CAD build for the part. Positions are in the model's coordinates, mm. A direction names the side the tool comes from. Give positions to 0.01 mm unless a question says otherwise; leave off trailing zeros. Order: outer loops, then holes, each group sorted by start corner. A loop starts at its lowest first (then second) coordinate and runs counter-clockwise, first axis right, second up.
Item 1: Flat gauge pins, fed straight in: P1, Ø1, axis at x = -50.5, z = 1, coming from the -Y side; P2, Ø5, axis at x = -38, y = -9, coming from the -Z side; P3, Ø0.9, axis at x = -24.5, z = 1, coming from the -Y side. Where does each tip first touch, or does it go through?
Item 2: Band-saw the part on B-B on y = -8.5. Give the cut face in (x, z), plus the area to 3 significant figures.
Item 3: Band-saw the part on D-D on y = -0.5. Give the cut face in (x, z), plus the area to 3 significant figures.
Item 4: Band-saw the part on A-A on x = -39. Give the cut face in (y, z), plus the area to 3 significant figures.
Item 5: Band-saw the part on C-C on z = 1.6. Give the cut face in (x, y), plus the area to 3 significant figures.
Item 6: Which spindle directions (+Z, -Z, +X, -X, +Y, -Y) get a long thin tool onto all of the face, cutting with end or side? Do faces 1 (the cylindrical face through (-51.5, -0.07, 1.48)), 2 (the flat face through (-30, 4.5, 1)), 3 (the flat face through (-30, -4.5, 1)). Say none if no direction does.
Item 7: Two-plate mould, pull along Y, no slides. Class faces 4 (the flat face through (-56.623, -1.288, 1.479)), 5 (the cylindrical face through (-40.2, -0.9, 1.5)), 6 (the cylindrical face through (-7.5, 0.1, 1.5)), 7 (the cylindrical face through (-59.277, -7.844, 1.479)): released by +Y, released by -Y, zero draft, split by the parting line, or undercut.
Item 8: Wall check: L1, parallel to Y at x = -39, z = 1.1; L2, parallel to Y at x = -29, z = 1.85; L3, parallel to X at y = -7, z = 2.35. Give the ranges that are in metal, low to high.
Autodesk Inventor part; units mm, degrees
ref_plane "YZ Plane" through (0, 0, 0) normal (1, 0, 0) x (0, 1, 0)
ref_plane "XZ Plane" through (0, 0, 0) normal (0, 1, 0) x (-1, 0, 0)
ref_plane "XY Plane" through (0, 0, 0) normal (0, 0, 1) x (1, 0, 0)
sketch "スケッチ1" plane through (0, 0, 0) normal (0, 0, 1) x (1, 0, 0)
  circle A0 centre (-55, 0) radius 8.025 construction
  circle A1 centre (0, 0) radius 1.25 construction
  arc A2 (-44.5788, 6) -> (-63.6661, 8.3366) centre (-55, 0) ccw construction
  line L0 (-63.6661, 8.3366) -> (-109.1623, -38.9576) construction
  line L1 (-102.7709, -46.5745) -> (-48.2949, -9.9821) construction
  arc A3 (-48.2949, -9.9821) -> (-44.5788, -6) centre (-55, 0) ccw construction
  line L2 (-44.5788, -6) -> (-5.2915, -6) construction
  arc A4 (-5.2915, -6) -> (-5.2915, 6) centre (0, 0) ccw construction
  line L3 (-5.2915, 6) -> (-44.5788, 6) construction
  circle A5 centre (0, 0) radius 1.5
  circle A6 centre (-30, 0) radius 1.5
  circle A7 centre (-12, 0) radius 1.5
  circle A8 centre (-21, 0) radius 1.5
  line L4 (-30, 0) -> (0, 0)
  line L5 (-30, 0) -> (-50, 0)
  line L6 (-50, 0) -> (-30, 0)
  circle A9 centre (-50, 0) radius 1.5
  circle A10 centre (-50, 0) radius 4.025 construction
  circle A11 centre (-50, 0) radius 7.125 construction
  circle A12 centre (-57.7782, -7.7782) radius 1.5
  circle A13 centre (-57.7782, -7.7782) radius 3 construction
  line L7 (-50, 0) -> (-57.7782, -7.7782) construction
  line L8 (-53.1753, 3.2604) -> (-60.169, -5.9659)
  line L9 (-55.3874, -9.5904) -> (-46.209, 2.5181)
  arc A14 (-46.209, 2.5181) -> (-53.1753, 3.2604) centre (-50, 0) ccw
  arc A15 (-60.169, -5.9659) -> (-55.3874, -9.5904) centre (-57.7782, -7.7782) ccw
  line L10 (-50, 0) -> (0, 0) construction
  line L11 (-50, -4.5) -> (0, -4.5)
  line L12 (0, 4.5) -> (-50, 4.5)
  arc A16 (-50, 4.5) -> (-50, -4.5) centre (-50, 0) ccw
  arc A17 (0, -4.5) -> (0, 4.5) centre (0, 0) ccw
  line L13 (-57.7782, -10.7782) -> (-54.9706, -10.7782)
  line L14 (-54.9706, -10.7782) -> (-48.1997, -4.5)
  line L15 (-50, 0) -> (-57.7782, -7.7782)
  circle A18 centre (-12, 0) radius 4.5
  point P0 (-53.8891, -3.8891)
  point P1 (-25, 0)
  point P2 (-48.7574, -3)
  point P3 (-49.3198, 4.5)
  point P4 (-53.5862, 2.7184)
  point P5 (-51.3675, -4.2872)
  point P6 (-12, -4.5)
  point P7 (-12, 4.5)
  dimension "d25" = 3
  dimension "d26" = 0
  dimension "d0" = 20
  dimension "d2" = 3
  dimension "d3" = 8.05
  dimension "d4" = 3.1
  dimension "d5" = 30
  dimension "d6" = 3
  dimension "d7" = 3
  dimension "d8" = 3
  dimension "d9" = 3
  dimension "d11" = 9
  dimension "d13" = 3
  dimension "d14" = 6
  dimension "d15" = 6
  dimension "d16" = 9
  dimension "d21" = 135
  dimension "d22" = 10
  dimension "d30" = 9
  dimension "d31" = 11
extrude "押し出し1" add sketch "スケッチ1" along normal blind 3 contours L4 A8 A18 L11 A16 L9 L5 A6 | A6 L5 L9 A14 L12 A18 L4 A8 | L9 A9 L5 | L5 A9 L15 A16 L12 A14 L9 | L9 A16 L15 A9 | A18 L4 A7 | L4 A7 A18 | A16 L11 L14 L13 A15 L9 | L9 A15 L8 A16 | L12 A16 L8 A14
fillet "フィレット1" radius 1.05 1 edges at (-48.1997, -4.5, 1.5)
sketch "スケッチ2" plane through (0, 0, 3) normal (0, 0, 1) x (1, 0, 0)
  arc A0 (-60.7927, -6.5251) -> (-59.7797, -5.8711) centre (-60.7525, -5.4759) ccw
  arc A1 (-55.3849, -4.4725) -> (-59.7797, -5.8711) centre (-57.0004, -7.0004) ccw
  arc A2 (-55.3849, -4.4725) -> (-43.7567, 3.1657) centre (-50, 0) ccw
  arc A3 (-44.0452, 4.6286) -> (-43.7567, 3.1657) centre (-43.1001, 4.055) ccw
  line L0 (-44.0452, 4.6286) -> (-41.5381, 8.9709)
  arc A4 (-41.5381, 8.9709) -> (-46.5567, 11.6351) centre (-44, 10.3923) ccw
  line L1 (-46.5567, 11.6351) -> (-49.0637, 7.2927)
  arc A5 (-50.5985, 6.9744) -> (-49.0637, 7.2927) centre (-49.9731, 7.8177) ccw
  arc A6 (-50.5985, 6.9744) -> (-50.2678, 6.9949) centre (-50, 0) ccw
  circle A7 centre (-50, 0) radius 4.025
  circle A8 centre (-50, 0) radius 1.5
  circle A9 centre (-39, 0) radius 4
  line L2 (-50, 0) -> (-38.3804, 0)
  circle A10 centre (-39, 0) radius 1.5
  circle A11 centre (-30, 0) radius 1.5
  point P0 (0, 0)
  point P1 (-43.3711, 2.3255)
  point P2 (-43, 0)
  point P3 (-49.3534, 6.9701)
  point P4 (-44.1966, 3.9141)
  point P5 (-43.7567, 3.1657)
  dimension "d23" = 12
  dimension "d24" = 8
  dimension "d27" = 3
  dimension "d28" = 9
  dimension "d29" = 7
extrude "押し出し2" cut sketch "スケッチ2" against normal blind 3 contours A10
properties part number "中間節アーム先端締結パーツ内" material "アルミニウム 7075"
The answers:
1. P1: stops at y = -7.1
1. P2: passes through
1. P3: stops at y = -4.5
2. outline: (-60.69, 0) - (-59.09, 0) - (-59.09, 3) - (-60.69, 3) - close; (-56.46, 0) - (-52.51, 0) - (-52.51, 3) - (-56.46, 3) - close
2. area: 16.6 mm2
3. outline: (-56.03, 0) - (-51.41, 0) - (-51.41, 3) - (-56.03, 3) - close; (-48.59, 0) - (-40.41, 0) - (-40.41, 3) - (-48.59, 3) - close; (-37.59, 0) - (-31.41, 0) - (-31.41, 3) - (-37.59, 3) - close; (-28.59, 0) - (-22.41, 0) - (-22.41, 3) - (-28.59, 3) - close; (-19.59, 0) - (-13.41, 0) - (-13.41, 3) - (-19.59, 3) - close; (-10.59, 0) - (-7.53, 0) - (-7.53, 3) - (-10.59, 3) - close
3. area: 103 mm2
4. outline: (-4.5, 0) - (-1.5, 0) - (-1.5, 3) - (-4.5, 3) - close; (1.5, 0) - (4.5, 0) - (4.5, 3) - (1.5, 3) - close
4. area: 18.0 mm2
5. outline: (-60.17, -5.97) arc R3 ccw to (-57.78, -10.78) - (-54.97, -10.78) - (-48.5, -4.78) arc R1.05 cw to (-47.79, -4.5) - (-12, -4.5) arc R4.5 ccw to (-12, 4.5) - (-49.32, 4.5) arc R4.55 ccw to (-53.18, 3.26) - close; hole circle Ø3 at (-57.78, -7.78); hole circle Ø3 at (-50, 0); hole circle Ø3 at (-39, 0); hole circle Ø3 at (-30, 0); hole circle Ø3 at (-21, 0); hole circle Ø3 at (-12, 0)
5. area: 435 mm2
6. face 1: +Z, -Z
6. face 2: +Z, -Z, +X, +Y
6. face 3: +Z, -Z, +X, -Y
7. face 4: released by +Y
7. face 5: undercut
7. face 6: split by the parting line
7. face 7: undercut
8. L1: y = -4.5 to -1.5, 1.5 to 4.5
8. L2: y = -4.5 to -1.12, 1.12 to 4.5
8. L3: x = -60.68 to -59.06, -56.5 to -50.9
